Model file for the job. Use its own axes, mm. A direction names the side the tool comes from. Round coordinates to 2 decimals unless told otherwise and drop trailing zeros. Order: outer loops, then holes, each group sorted by start corner. A loop starts at its lowest first (then second) coordinate and runs counter-clockwise, first axis right, second up. Notation, with made-up numbers: (88, 11) - (127, 11) arc R23 cw to (127, 29) - close; hole circle Ø6 at (35, -7). An arc over 180 degrees is marked (long way). Write item = value, one per line.
```python
from build123d import *

# Parameters (mm, degrees)
SKETCH1_W                = 30
SKETCH1_H                = 30
BASE_FLANGE1_DEPTH       = 1.5
EDGE_FLANGE1_DEPTH       = 30
EDGE_FLANGE1_START       = -1.5
EDGE_FLANGE1_PROFILE_R   = 1.5
EDGE_FLANGE1_PROFILE_R_2 = 3.6
EDGE_FLANGE1_FLAT_DEPTH  = 1.5


# Sheet-metal steps are written as plain solids
with BuildPart() as part:
    # Sketch1 → Base-Flange1 (new body)
    with BuildSketch(Plane(origin=(0, 0, 0), x_dir=(1, 0, 0), z_dir=(0, 1, 0))):
        Rectangle(SKETCH1_W, SKETCH1_H)
        with BuildLine():
            Line((-8.617716364, 6), (-8.617716364, -8))
            ThreePointArc((-8.617716364, -8), (-10.617716364, -10), (-12.617716364, -8))
            Line((-12.617716364, -8), (-12.617716364, 6))
            ThreePointArc((-12.617716364, 6), (-10.617716364, 8), (-8.617716364, 6))
        make_face(mode=Mode.SUBTRACT)
        with BuildLine():
            Line((8.617716364, 6), (8.617716364, -8))
            ThreePointArc((8.617716364, -8), (10.617716364, -10), (12.617716364, -8))
            Line((12.617716364, -8), (12.617716364, 6))
            ThreePointArc((12.617716364, 6), (10.617716364, 8), (8.617716364, 6))
        make_face(mode=Mode.SUBTRACT)
        with BuildLine():
            Line((-3, 8), (3, 8))
            ThreePointArc((3, 8), (5, 6), (3, 4))
            Line((3, 4), (-3, 4))
            ThreePointArc((-3, 4), (-5, 6), (-3, 8))
        make_face(mode=Mode.SUBTRACT)
        with BuildLine():
            Line((-3, -8), (3, -8))
            ThreePointArc((3, -8), (5, -6), (3, -4))
            Line((3, -4), (-3, -4))
            ThreePointArc((-3, -4), (-5, -6), (-3, -8))
        make_face(mode=Mode.SUBTRACT)
    extrude(amount=-BASE_FLANGE1_DEPTH)

    # Edge-Flange1 bend section (across the edge) → Edge-Flange1 (add)
    with BuildSketch(Plane(origin=(-15, 0, 15.7366), x_dir=(0, 0, -1), z_dir=(1, 0, 0))):
        with BuildLine():
            Line((-1.5, 0.7366), (0, 0.7366))
            ThreePointArc((0, 0.7366), (0.215745145, 0.215745145), (0.7366, 0))
            Line((0.7366, 0), (0.7366, -1.5))
            ThreePointArc((0.7366, -1.5), (-0.844915027, -0.844915027), (-1.5, 0.7366))
        make_face()
    extrude(amount=EDGE_FLANGE1_DEPTH)

    # Edge-Flange1 profile (on flange) → Edge-Flange1 flat (add)
    with BuildSketch(Plane(origin=(0, 0, 15.7366), x_dir=(-1, 0, 0), z_dir=(0, 0, -1)).offset(EDGE_FLANGE1_START)):
        with BuildLine():
            ThreePointArc((15, 20.067164179), (0, 33.5), (-15, 20.067164179))
            Line((-15, 20.067164179), (-15, 0.7366))
            Line((-15, 0.7366), (15, 0.7366))
            Line((15, 0.7366), (15, 20.067164179))
        make_face()
        with Locations((8.5, 16.75)):
            Circle(EDGE_FLANGE1_PROFILE_R, mode=Mode.SUBTRACT)
        with Locations((0, 16.75)):
            Circle(EDGE_FLANGE1_PROFILE_R_2, mode=Mode.SUBTRACT)
        with Locations((-8.5, 16.75)):
            Circle(EDGE_FLANGE1_PROFILE_R, mode=Mode.SUBTRACT)
    extrude(amount=EDGE_FLANGE1_FLAT_DEPTH)


solid = part.part
```
1) 3-axis set-ups, long thin cutter, end or side, ignore diameter. For faces 1 (the face through (0, -1, 8)), 2 (the face through (0, -1, -15)): which of +Z, -Z, +X, -X, +Y, -Y reach the whole face in a straight line?
Conclusion:
face_1 = +Y, -Y
face_2 = -Z, +X, -X, +Y, -Y
2) Flat gauge pins, fed straight in: pin 1 Ø10 at (x, y) = (-4, 17) entering from -Z; pin 2 Ø3 at (x, z) = (-10, -10.5) entering from +Y; pin 3 Ø0.8 at (x, y) = (1, -0.5) entering from +Z. Where does each tip first touch, or does it go through?
Conclusion:
pin_1 = 15.74
pin_2 = 0
pin_3 = 17.07
3) Wall check: line 1 along X through (y, z) = (16, 16); line 2 along Y through (x, z) = (-4, 1.5); line 3 along Z through (x, y) = (-10, 1.5). Give the ranges that are in metal, low to high.
Conclusion:
line_1 = -15 to -9.8, -7.2 to -3.52, 3.52 to 7.2, 9.8 to 15
line_2 = -1.5 to 0
line_3 = 15.74 to 17.24
4) Cut at B-B (y = 16.75). Write the cut outline in (x, z), and give its area (3 significant figures).
Conclusion:
outline = (-15, 15.74) - (-10, 15.74) - (-10, 17.24) - (-15, 17.24) - close; (-7, 15.74) - (-3.6, 15.74) - (-3.6, 17.24) - (-7, 17.24) - close; (3.6, 15.74) - (7, 15.74) - (7, 17.24) - (3.6, 17.24) - close; (10, 15.74) - (15, 15.74) - (15, 17.24) - (10, 17.24) - close
area = 25.2 mm^2
5) Mould opens along Y. For faces 3 (the face through (0, 0, 0)), 4 (the face through (-0.21, -0.862, 16.564)), 5 (the face through (0, -1, -8)), 6 (the face through (0.78, 13.236, 16.497)) say: +Y half, -Y half, draft (parallel to the pull), parting line (faces both ways), or undercut.
Conclusion:
face_3 = +Y half
face_4 = -Y half
face_5 = draft
face_6 = undercut
6) Cut at C-C (z = 2). Write the cut outline in (x, y).
Conclusion:
outline = (-15, -1.5) - (-12.62, -1.5) - (-12.62, 0) - (-15, 0) - close; (-8.62, -1.5) - (8.62, -1.5) - (8.62, 0) - (-8.62, 0) - close; (12.62, -1.5) - (15, -1.5) - (15, 0) - (12.62, 0) - close
7) Cut at D-D (y = 7). Write the cut outline in (x, z).
Conclusion:
outline = (-15, 15.74) - (15, 15.74) - (15, 17.24) - (-15, 17.24) - close
8) Cut at A-A (z = 6). Write the cut outline in (x, y), and give its area (3 significant figures).
Conclusion:
outline = (-15, -1.5) - (-12.62, -1.5) - (-12.62, 0) - (-15, 0) - close; (-8.62, -1.5) - (-5, -1.5) - (-5, 0) - (-8.62, 0) - close; (5, -1.5) - (8.62, -1.5) - (8.62, 0) - (5, 0) - close; (12.62, -1.5) - (15, -1.5) - (15, 0) - (12.62, 0) - close
area = 18.0 mm^2
